Here's how the part is built. I have some questions about the finished solid (model axes, mm). A direction names the side the tool comes from. Round coordinates to 2 decimals unless told otherwise and drop trailing zeros. Write each loop counter-clockwise with the first axis right and the second up, starting at its lowest first coordinate (ties: lowest second). Pieces come first, ordered by that corner, then holes. Notation, with made-up numbers: M 71.25,20.25 L 127.25,20.25 A17 cw 127.25,33.25 Z; hole C -15.75,83 d8. An arc over 180 degrees is marked long. Write item = value, one per line. Start each with the question number.
(1) I want a section at B-B (z = -363). List the corners of the cut face in (x, y) for me.
(2) Will these pins go through, and if not, where does the flat tip stop? pin 1 Ø12 at (x, y) = (398.5, -515) entering from +Z; pin 2 Ø5 at (x, z) = (280.5, -420.5) entering from +Y.
(3) I want a section at A-A (x = -273). List the corners of the cut face in (y, z) for me, and give its area (3 significant figures).
(4) I need wall thicknesses on line 1 along X through (y, z) = (-607, 136); line 2 along Z through (x, y) = (1, -737); line 3 along Y through (x, z) = (-282.5, -151). Which ranges of each line are inside material? Lowest first, please.
(5) On a 3-axis mill with a long thin cutter (end or side, diameter ignored), from which of +Z, -Z, +X, -X, +Y, -Y can I reach the whole of each face in a straight line? I mean faces 1 (the flat face through (0.444, -545, -3)), 2 (the flat face through (-257, -254, -3)), 3 (the flat face through (380, -508, -386)). Say none if no direction works.
(6) I want a section at D-D (y = -476.5). List the corners of the cut face in (x, z) for me, and give its area (3 significant figures).
(7) I want a section at C-C (y = -612.5). List the corners of the cut face in (x, z) for me.
```python
from build123d import *

# Parameters (mm, degrees)
F0_W      = 1016
F0_H      = 762
F1_DEPTH  = 1016
F2_W      = 254
F2_H      = 508
F3_DEPTH  = 1016
F6_DEPTH  = 508
F7_DEPTH  = 25
F9_DEPTH  = 254
F11_DEPTH = 762
F12_SIZE  = 254


with BuildPart() as f1:
    # F0 (on Front) → F1 (new body)
    with BuildSketch(Plane.XZ):
        with Locations((0.4440769553, -133.8159580914)):
            Rectangle(F0_W, F0_H)
    extrude(amount=F1_DEPTH)

    # F2 (on face) → F3 (cut)
    with BuildSketch(Plane.XY.offset(247.1840419086)):
        with Locations((381.4440769553, -254)):
            Rectangle(F2_W, F2_H)
    extrude(amount=-F3_DEPTH, mode=Mode.SUBTRACT)

    # F4 (on face) → F6 (cut)
    with BuildSketch(Plane.XY.offset(247.1840419086)):
        Polygon((0.4440769553, -254), (0.4440769553, -1016), (508.4440769553, -1016), (508.4440769553, -508), (254.4440769553, -508), (254.4440769553, 0), (-507.5559230447, 0), (-507.5559230447, -254), align=None)
    extrude(amount=-F6_DEPTH, mode=Mode.SUBTRACT)

    # F10 (on face) → F11 (cut)
    with BuildSketch(Plane(origin=(-507.5559230447, 0, 0), x_dir=(0, -1, 0), z_dir=(-1, 0, 0))):
        Polygon((1016, -102.9850542545), (1016, 247.1840419086), (635, 247.1840419086), align=None)
    extrude(amount=-F11_DEPTH, mode=Mode.SUBTRACT)

    # F12
    f12_edges = [f1.edges().sort_by_distance(p)[0] for p in [
        (508.444077, -1016, -387.815958),
    ]]
    chamfer(f12_edges, length=F12_SIZE)


with BuildPart() as f7:
    # F5 (on face) → F7 (new body)
    with BuildSketch(Plane.XY.offset(247.1840419086)):
        Polygon((254.4440769553, 0), (-506.6555738449, 0), (-506.6555738449, -254), (0.4440769553, -254), (0.4440769553, -1016), (508.4440769553, -1016), (508.4440769553, -508), (254.4440769553, -508), align=None)
    extrude(amount=F7_DEPTH)

    # F8 (on face) → F9 (cut)
    with BuildSketch(Plane.XY.offset(272.1840419086)):
        Polygon((-506.6555738449, -254), (0.4440769553, -254), (0.4440769553, -1016), (508.4440769553, -1016), (508.4440769553, -508), (254.4440769553, -508), (254.4440769553, 0), (-506.6555738449, 0), align=None)
    extrude(amount=-F9_DEPTH, mode=Mode.SUBTRACT)


solid = f1.part
```
Returned:
q1.outline = M -507.56,-1016 L 254.44,-1016 L 508.44,-762 L 508.44,-508 L 254.44,-508 L 254.44,0 L -507.56,0 Z
q2.pin_1 = -260.82
q2.pin_2 = -508
q3.outline = M -1016,-514.82 L 0,-514.82 L 0,-260.82 L -254,-260.82 L -254,247.18 L -635,247.18 L -1016,-102.99 Z
q3.area = 578,000 mm²
q4.line_1 = -507.56 to 0.44
q4.line_2 = -514.82 to -260.82
q4.line_3 = -1016 to -254
q5.face_1 = +Z, +X, +Y, -Y
q5.face_2 = +Z, +X, -X, +Y
q5.face_3 = +Z, -Z, +X, +Y
q6.outline = M -507.56,-514.82 L 254.44,-514.82 L 254.44,-260.82 L 0.44,-260.82 L 0.44,247.18 L -507.56,247.18 Z
q6.area = 452,000 mm²
q7.outline = M -507.56,-514.82 L 508.44,-514.82 L 508.44,-260.82 L 0.44,-260.82 L 0.44,247.18 L -507.56,247.18 Z
